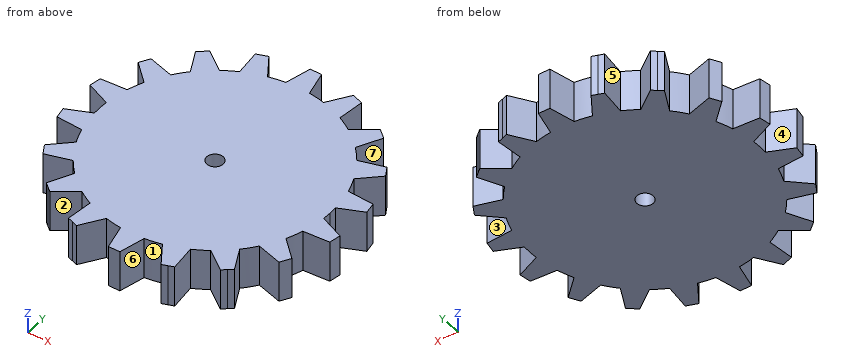
from build123d import *

# Parameters (mm, degrees)
F0_R     = 1
F1_DEPTH = 5


with BuildPart() as f1:
    # F0 (on Top) → F1 (new body)
    with BuildSketch(Plane.XY):
        with BuildLine():
            ThreePointArc((13.964093, -1.002049), (13.99102, -0.501346), (14, 0))
            ThreePointArc((14, 0), (13.99102, 0.501346), (13.964093, 1.002049))
            ThreePointArc((13.964093, 1.002049), (13.787309, 2.431074), (13.464676, 3.834383))
            ThreePointArc((13.464676, 3.834383), (13.155697, 4.788282), (12.779234, 5.717619))
            ThreePointArc((12.779234, 5.717619), (12.124356, 7), (11.341221, 8.208332))
            ThreePointArc((11.341221, 8.208332), (10.724622, 8.999027), (10.053011, 9.74356))
            ThreePointArc((10.053011, 9.74356), (8.999027, 10.724622), (7.849846, 11.592235))
            ThreePointArc((7.849846, 11.592235), (7, 12.124356), (6.114247, 12.594284))
            ThreePointArc((6.114247, 12.594284), (4.788282, 13.155697), (3.411665, 13.577943))
            ThreePointArc((3.411665, 13.577943), (2.431074, 13.787309), (1.438014, 13.925951))
            ThreePointArc((1.438014, 13.925951), (0, 14), (-1.438014, 13.925951))
            ThreePointArc((-1.438014, 13.925951), (-2.431074, 13.787309), (-3.411665, 13.577943))
            ThreePointArc((-3.411665, 13.577943), (-4.788282, 13.155697), (-6.114247, 12.594284))
            ThreePointArc((-6.114247, 12.594284), (-7, 12.124356), (-7.849846, 11.592235))
            ThreePointArc((-7.849846, 11.592235), (-8.999027, 10.724622), (-10.053011, 9.74356))
            ThreePointArc((-10.053011, 9.74356), (-10.724622, 8.999027), (-11.341221, 8.208332))
            ThreePointArc((-11.341221, 8.208332), (-12.124356, 7), (-12.779234, 5.717619))
            ThreePointArc((-12.779234, 5.717619), (-13.155697, 4.788282), (-13.464676, 3.834383))
            ThreePointArc((-13.464676, 3.834383), (-13.787309, 2.431074), (-13.964093, 1.002049))
            ThreePointArc((-13.964093, 1.002049), (-14, 0), (-13.964093, -1.002049))
            ThreePointArc((-13.964093, -1.002049), (-13.787309, -2.431074), (-13.464676, -3.834383))
            ThreePointArc((-13.464676, -3.834383), (-13.155697, -4.788282), (-12.779234, -5.717619))
            ThreePointArc((-12.779234, -5.717619), (-12.124356, -7), (-11.341221, -8.208332))
            ThreePointArc((-11.341221, -8.208332), (-10.724622, -8.999027), (-10.053011, -9.74356))
            ThreePointArc((-10.053011, -9.74356), (-8.999027, -10.724622), (-7.849846, -11.592235))
            ThreePointArc((-7.849846, -11.592235), (-7, -12.124356), (-6.114247, -12.594284))
            ThreePointArc((-6.114247, -12.594284), (-4.788282, -13.155697), (-3.411665, -13.577943))
            ThreePointArc((-3.411665, -13.577943), (-2.431074, -13.787309), (-1.438014, -13.925951))
            ThreePointArc((-1.438014, -13.925951), (0, -14), (1.438014, -13.925951))
            ThreePointArc((1.438014, -13.925951), (2.431074, -13.787309), (3.411665, -13.577943))
            ThreePointArc((3.411665, -13.577943), (4.788282, -13.155697), (6.114247, -12.594284))
            ThreePointArc((6.114247, -12.594284), (7, -12.124356), (7.849846, -11.592235))
            ThreePointArc((7.849846, -11.592235), (8.999027, -10.724622), (10.053011, -9.74356))
            ThreePointArc((10.053011, -9.74356), (10.724622, -8.999027), (11.341221, -8.208332))
            ThreePointArc((11.341221, -8.208332), (12.124356, -7), (12.779234, -5.717619))
            ThreePointArc((12.779234, -5.717619), (13.155697, -4.788282), (13.464676, -3.834383))
            ThreePointArc((13.464676, -3.834383), (13.787309, -2.431074), (13.964093, -1.002049))
        make_face()
        Circle(F0_R, mode=Mode.SUBTRACT)
        with BuildLine():
            Line((15.072432, -7.893782), (12.779234, -5.717619))
            ThreePointArc((12.779234, -5.717619), (12.124356, -7), (11.341221, -8.208332))
            Line((11.341221, -8.208332), (14.372432, -9.106218))
            Line((14.372432, -9.106218), (14.722432, -8.5))
            Line((14.722432, -8.5), (15.072432, -7.893782))
        make_face()
        with BuildLine():
            Line((0.7, -17), (1.438014, -13.925951))
            ThreePointArc((1.438014, -13.925951), (0, -14), (-1.438014, -13.925951))
            Line((-1.438014, -13.925951), (-0.7, -17))
            Line((-0.7, -17), (0, -17))
            Line((0, -17), (0.7, -17))
        make_face()
        with BuildLine():
            Line((-10.391158, -13.472707), (-7.849846, -11.592235))
            ThreePointArc((-7.849846, -11.592235), (-8.999027, -10.724622), (-10.053011, -9.74356))
            Line((-10.053011, -9.74356), (-11.46362, -12.572804))
            Line((-11.46362, -12.572804), (-10.927389, -13.022756))
            Line((-10.927389, -13.022756), (-10.391158, -13.472707))
        make_face()
        with BuildLine():
            Line((11.46362, -12.572804), (10.053011, -9.74356))
            ThreePointArc((10.053011, -9.74356), (8.999027, -10.724622), (7.849846, -11.592235))
            Line((7.849846, -11.592235), (10.391158, -13.472707))
            Line((10.391158, -13.472707), (10.927389, -13.022756))
            Line((10.927389, -13.022756), (11.46362, -12.572804))
        make_face()
        with BuildLine():
            Line((-5.156558, -16.214189), (-3.411665, -13.577943))
            ThreePointArc((-3.411665, -13.577943), (-4.788282, -13.155697), (-6.114247, -12.594284))
            Line((-6.114247, -12.594284), (-6.472127, -15.73536))
            Line((-6.472127, -15.73536), (-5.814342, -15.974775))
            Line((-5.814342, -15.974775), (-5.156558, -16.214189))
        make_face()
        with BuildLine():
            ThreePointArc((13.464676, 3.834383), (13.787309, 2.431074), (13.964093, 1.002049))
            Line((13.964093, 1.002049), (16.863286, 2.262654))
            Line((16.863286, 2.262654), (16.741732, 2.952019))
            Line((16.741732, 2.952019), (16.620178, 3.641384))
            Line((16.620178, 3.641384), (13.464676, 3.834383))
        make_face()
        with BuildLine():
            Line((16.863286, -2.262654), (13.964093, -1.002049))
            ThreePointArc((13.964093, -1.002049), (13.787309, -2.431074), (13.464676, -3.834383))
            Line((13.464676, -3.834383), (16.620178, -3.641384))
            Line((16.620178, -3.641384), (16.741732, -2.952019))
            Line((16.741732, -2.952019), (16.863286, -2.262654))
        make_face()
        with BuildLine():
            Line((6.472127, -15.73536), (6.114247, -12.594284))
            ThreePointArc((6.114247, -12.594284), (4.788282, -13.155697), (3.411665, -13.577943))
            Line((3.411665, -13.577943), (5.156558, -16.214189))
            Line((5.156558, -16.214189), (5.814342, -15.974775))
            Line((5.814342, -15.974775), (6.472127, -15.73536))
        make_face()
        with BuildLine():
            ThreePointArc((-1.438014, 13.925951), (0, 14), (1.438014, 13.925951))
            Line((1.438014, 13.925951), (0.7, 17))
            Line((0.7, 17), (0, 17))
            Line((0, 17), (-0.7, 17))
            Line((-0.7, 17), (-1.438014, 13.925951))
        make_face()
        with BuildLine():
            ThreePointArc((3.411665, 13.577943), (4.788282, 13.155697), (6.114247, 12.594284))
            Line((6.114247, 12.594284), (6.472127, 15.73536))
            Line((6.472127, 15.73536), (5.814342, 15.974775))
            Line((5.814342, 15.974775), (5.156558, 16.214189))
            Line((5.156558, 16.214189), (3.411665, 13.577943))
        make_face()
        with BuildLine():
            ThreePointArc((11.341221, 8.208332), (12.124356, 7), (12.779234, 5.717619))
            Line((12.779234, 5.717619), (15.072432, 7.893782))
            Line((15.072432, 7.893782), (14.722432, 8.5))
            Line((14.722432, 8.5), (14.372432, 9.106218))
            Line((14.372432, 9.106218), (11.341221, 8.208332))
        make_face()
        with BuildLine():
            ThreePointArc((-6.114247, 12.594284), (-4.788282, 13.155697), (-3.411665, 13.577943))
            Line((-3.411665, 13.577943), (-5.156558, 16.214189))
            Line((-5.156558, 16.214189), (-5.814342, 15.974775))
            Line((-5.814342, 15.974775), (-6.472127, 15.73536))
            Line((-6.472127, 15.73536), (-6.114247, 12.594284))
        make_face()
        with BuildLine():
            ThreePointArc((-12.779234, 5.717619), (-12.124356, 7), (-11.341221, 8.208332))
            Line((-11.341221, 8.208332), (-14.372432, 9.106218))
            Line((-14.372432, 9.106218), (-14.722432, 8.5))
            Line((-14.722432, 8.5), (-15.072432, 7.893782))
            Line((-15.072432, 7.893782), (-12.779234, 5.717619))
        make_face()
        with BuildLine():
            ThreePointArc((7.849846, 11.592235), (8.999027, 10.724622), (10.053011, 9.74356))
            Line((10.053011, 9.74356), (11.46362, 12.572804))
            Line((11.46362, 12.572804), (10.927389, 13.022756))
            Line((10.927389, 13.022756), (10.391158, 13.472707))
            Line((10.391158, 13.472707), (7.849846, 11.592235))
        make_face()
        with BuildLine():
            ThreePointArc((-10.053011, 9.74356), (-8.999027, 10.724622), (-7.849846, 11.592235))
            Line((-7.849846, 11.592235), (-10.391158, 13.472707))
            Line((-10.391158, 13.472707), (-10.927389, 13.022756))
            Line((-10.927389, 13.022756), (-11.46362, 12.572804))
            Line((-11.46362, 12.572804), (-10.053011, 9.74356))
        make_face()
        with BuildLine():
            ThreePointArc((-13.964093, 1.002049), (-13.787309, 2.431074), (-13.464676, 3.834383))
            Line((-13.464676, 3.834383), (-16.620178, 3.641384))
            Line((-16.620178, 3.641384), (-16.741732, 2.952019))
            Line((-16.741732, 2.952019), (-16.863286, 2.262654))
            Line((-16.863286, 2.262654), (-13.964093, 1.002049))
        make_face()
        with BuildLine():
            Line((-16.620178, -3.641384), (-13.464676, -3.834383))
            ThreePointArc((-13.464676, -3.834383), (-13.787309, -2.431074), (-13.964093, -1.002049))
            Line((-13.964093, -1.002049), (-16.863286, -2.262654))
            Line((-16.863286, -2.262654), (-16.741732, -2.952019))
            Line((-16.741732, -2.952019), (-16.620178, -3.641384))
        make_face()
        with BuildLine():
            Line((-14.372432, -9.106218), (-11.341221, -8.208332))
            ThreePointArc((-11.341221, -8.208332), (-12.124356, -7), (-12.779234, -5.717619))
            Line((-12.779234, -5.717619), (-15.072432, -7.893782))
            Line((-15.072432, -7.893782), (-14.722432, -8.5))
            Line((-14.722432, -8.5), (-14.372432, -9.106218))
        make_face()
    extrude(amount=F1_DEPTH)


solid = f1.part
Verification items for the finished model (mm, model axes). Face numbers are marked on the shaded views. A direction names the side the tool comes from. Round coordinates to 2 decimals unless told otherwise and drop trailing zeros. Write each loop counter-clockwise with the first axis right and the second up, starting at its lowest first coordinate (ties: lowest second). Pieces come first, ordered by that corner, then holes.
(1) Section check B-B (x = 15.5). Enter the section's corners in (y, z).
Returned:
outline: (-3.71, 0) - (-1.67, 0) - (-1.67, 5) - (-3.71, 5) - close; (1.67, 0) - (3.71, 0) - (3.71, 5) - (1.67, 5) - close
(2) Section check A-A (x = 0). Enter the section's corners in (y, z).
Returned:
outline: (-17, 0) - (-1, 0) - (-1, 5) - (-17, 5) - close; (1, 0) - (17, 0) - (17, 5) - (1, 5) - close
(3) Material ranges on line 1 (X direction, y = 14, z = 3.65); line 2 (X direction, y = -15, z = 2.9); line 3 (Y direction, x = 11, z = 0.2), recorded low to high.
Returned:
line 1: x = -6.27 to -3.69, -1.42 to 1.42, 3.69 to 6.27
line 2: x = -6.39 to -4.35, -1.18 to 1.18, 4.35 to 6.39
line 3: y = -12.96 to -11.64, -8.66 to 8.66, 11.64 to 12.96
(4) Section check C-C (x = -12). Enter the section's corners in (y, z).
Returned:
outline: (-8.4, 0) - (8.4, 0) - (8.4, 5) - (-8.4, 5) - close
(5) Access from +Z, -Z, +X, -X, +Y, -Y to the whole of each face (thin tool, end or side, straight path). Record for the marked faces 5, 6 and 7.
Returned:
face 5: +Z, -Z
face 6: +Z, -Z, -Y
face 7: +Z, -Z, +X
(6) Mould release check, pull along X, two halves, no side actions. Record for the marked faces 1, 2, 3 and 4: pulls with the +X half, pulls with the -X half, needs draft (parallel to the pull), parting line crosses it, or undercut.
Returned:
face 1: undercut
face 2: undercut
face 3: pulls with the +X half
face 4: pulls with the -X half
(7) Depth check by flat-ended pin: pin 1 Ø3 at (y, z) = (-4.5, 3) entering from -X; pin 2 Ø1 at (x, z) = (-3, 2.5) entering from -Y (3 decimals); pin 3 Ø1.5 at (x, z) = (10, 0.5) entering from +Y; pin 4 Ø1.8 at (x, y) = (0, 0) entering from +Z. Enter the tip coordinate at first touch or a pass-through.
Returned:
pin 1: stops at x = -16.73
pin 2: stops at y = -13.775
pin 3: stops at y = 13.47
pin 4: passes through
